Check sheet for the modelled part. Datum: model origin and axes. Units: mm. Face numbers are marked on the shaded views. A direction names the side the tool comes from. Give positions to 0.01 mm unless a question says otherwise; leave off trailing zeros. Loops run counter-clockwise (first coordinate to the right, second up) from the corner with the lowest first, then second, coordinate; pieces in that order, holes last.
```python
from build123d import *

# Parameters (mm, degrees)
SKETCH2_R               = 2.5
CUT_EXTRUDE1_DEPTH      = 18
CUT_EXTRUDE1_DEPTH_BACK = 18


with BuildPart() as part:
    # Sketch1 → Revolve1 (revolve)
    with BuildSketch(Plane.XY):
        Polygon((0, 0), (20, 0), (20, -11), (400, -11), (400, -14), (20, -14), (20, -17), (0, -17), align=None)
    revolve(axis=Axis((0, 0, 0), (1, 0, 0)))

    # Sketch2 → Cut-Extrude1 (cut, two sides)
    with BuildSketch(Plane.XY) as cut_extrude1_sk:
        with Locations((392.5, 0)):
            Circle(SKETCH2_R)
    extrude(amount=CUT_EXTRUDE1_DEPTH, mode=Mode.SUBTRACT)
    extrude(cut_extrude1_sk.sketch, amount=-CUT_EXTRUDE1_DEPTH_BACK, mode=Mode.SUBTRACT)


solid = part.part
```
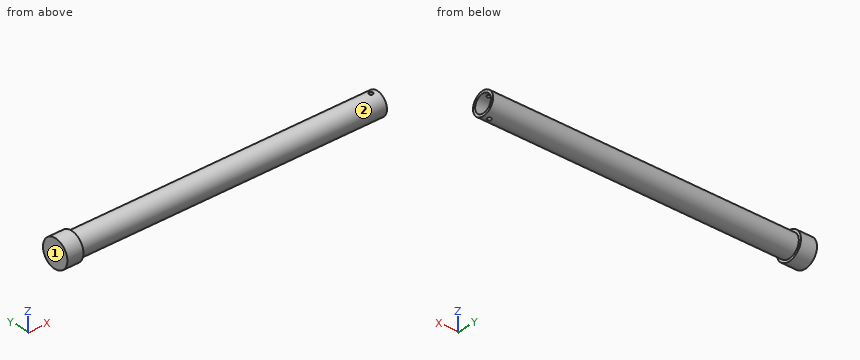
(1) Material ranges on line 1 (Y direction, x = 341, z = 1); line 2 (Z direction, x = 262, y = 0); line 3 (X direction, y = 1, z = 3), recorded low to high.
(2) Section check A-A on z = 0. Record the boundary of the cut face in (x, y), plus the area to 3 significant figures.
(3) Access from +Z, -Z, +X, -X, +Y, -Y to the whole of each face (thin tool, end or side, straight path). Record for the marked faces 1 and 2.
(4) Section check B-B on x = 69.5. Record the boundary of the cut face in (y, z), plus the area to 3 significant figures.
(5) Gauge pin test, flat ends, axial feed: pin 1 Ø13 at (y, z) = (0, 0) entering from +X; pin 2 Ø2 at (x, y) = (253, 1.5) entering from +Z; pin 3 Ø3 at (x, y) = (268, -4) entering from +Z (3 decimals); pin 4 Ø3 at (x, y) = (392.5, 0) entering from -Z. Record the tip position at first contact, or that the pin passes through.
Computed values:
1. line 1: y = -13.96 to -10.95, 10.95 to 13.96
1. line 2: z = -14 to -11, 11 to 14
1. line 3: x = 0 to 20
2. outline: (0, -17) - (20, -17) - (20, -14) - (400, -14) - (400, -11) - (20, -11) - (20, 11) - (400, 11) - (400, 14) - (20, 14) - (20, 17) - (0, 17) - close
2. area: 2,960 mm2
3. face 1: +Z, -Z, -X, +Y, -Y
3. face 2: +X
4. outline: circle Ø28 at (0, 0); hole circle Ø22 at (0, 0)
4. area: 236 mm2
5. pin 1: stops at x = 20
5. pin 2: stops at z = 13.99
5. pin 3: stops at z = 13.775
5. pin 4: passes through
